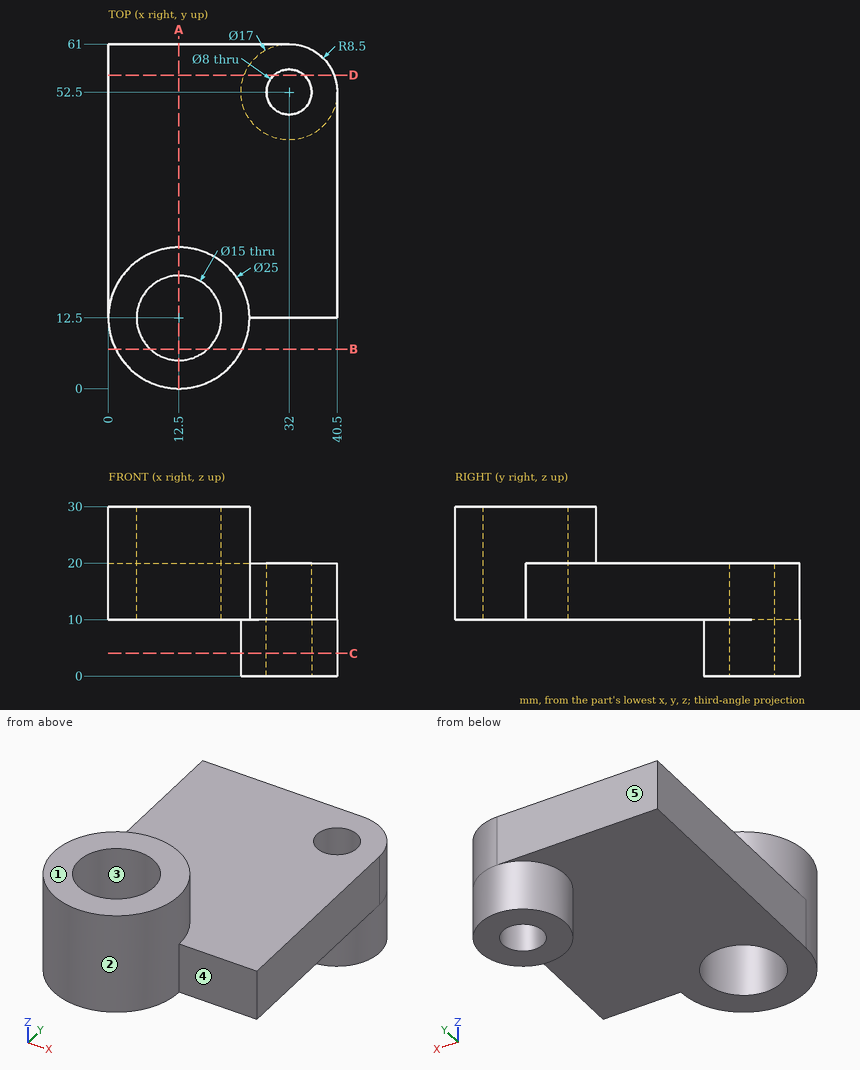
For this review, use the dimensioned drawing (mm, ordinates from the lowest corner) and the shaded views. A direction names the side the tool comes from. Round coordinates to 2 decimals unless told otherwise and drop trailing zeros. Write each loop counter-clockwise with the first axis right and the second up, starting at its lowest first coordinate (ties: lowest second). Pieces come first, ordered by that corner, then holes. Notation, with made-up numbers: (-34, 14) - (-20, 14) arc R12 ccw to (-20, 26) - close; hole circle Ø2 at (53.5, -38.75). An arc over 180 degrees is marked (long way). Answer as a JSON object with one key per item and string values.
1. We need section C-C on z = 4. Give the boundary of the cut face in (x, y), then the cut area to 3 significant figures.
Response values:
{"outline": "circle Ø17 at (32, 52.5); hole circle Ø8 at (32, 52.5)", "area": "177 mm2"}
2. Draft analysis for pull direction Y (two halves, no side actions). For the marked faces 1, 2 and 3, state which applies: +Y half, -Y half, draft (parallel to the pull), parting line (faces both ways), or undercut.
Response values:
{"face 1": "draft", "face 2": "parting line", "face 3": "undercut"}
3. Tool access review of the marked faces 4 and 5: name each direction out of +Z, -Z, +X, -X, +Y, -Y from which nothing blocks a thin tool from reaching the whole face with its end or side.
Response values:
{"face 4": "+Z, -Z, +X, -Y", "face 5": "+Z, -Z, +X, -X, +Y"}
4. We need section B-B on y = 7. Give the boundary of the cut face in (x, z).
Response values:
{"outline": "(1.28, 10) - (7.4, 10) - (7.4, 30) - (1.28, 30) - close; (17.6, 10) - (23.72, 10) - (23.72, 30) - (17.6, 30) - close"}
5. To check wall thickness, follow line 1 along Y through (x, z) = (12.5, 21); line 2 along Y through (x, z) = (32, 6.5); line 3 along X through (y, z) = (52.5, 8.25). State the ranges of each line that lie inside material, in increasing order.
Response values:
{"line 1": "y = 0 to 5, 20 to 25", "line 2": "y = 44 to 48.5, 56.5 to 61", "line 3": "x = 23.5 to 28, 36 to 40.5"}
6. We need section D-D on y = 55.5. Give the boundary of the cut face in (x, z).
Response values:
{"outline": "(0, 10) - (24.05, 10) - (24.05, 0) - (29.35, 0) - (29.35, 20) - (0, 20) - close; (34.65, 0) - (39.95, 0) - (39.95, 20) - (34.65, 20) - close"}
7. For pin 1 Ø1.5 at (x, y) = (20, 49.5) entering from +Z; pin 2 Ø11 at (x, z) = (29.5, 13.5) entering from -Y, all flat-tipped, find the tip position at first contact; note any pin that passes through.
Response values:
{"pin 1": "stops at z = 20", "pin 2": "stops at y = 7.6"}
8. We need section A-A on x = 12.5. Give the boundary of the cut face in (y, z), then the cut area to 3 significant figures.
Response values:
{"outline": "(0, 10) - (5, 10) - (5, 30) - (0, 30) - close; (20, 10) - (61, 10) - (61, 20) - (25, 20) - (25, 30) - (20, 30) - close", "area": "560 mm2"}
